Check sheet for the drawn part. Datum: minimum x, y, z corner. Units: mm. A direction names the side the tool comes from. Coordinates: 2 decimals unless noted, no trailing zeros. Loops run counter-clockwise (first coordinate to the right, second up) from the corner with the lowest first, then second, coordinate; pieces in that order, holes last. Notation, with made-up numbers: (-15.75, 70) - (12.25, 70) arc R28 cw to (12.25, 107) - close; hole circle Ø7 at (9.25, 83). An arc over 180 degrees is marked (long way). Write item = value, one per line. Start each with the question number.
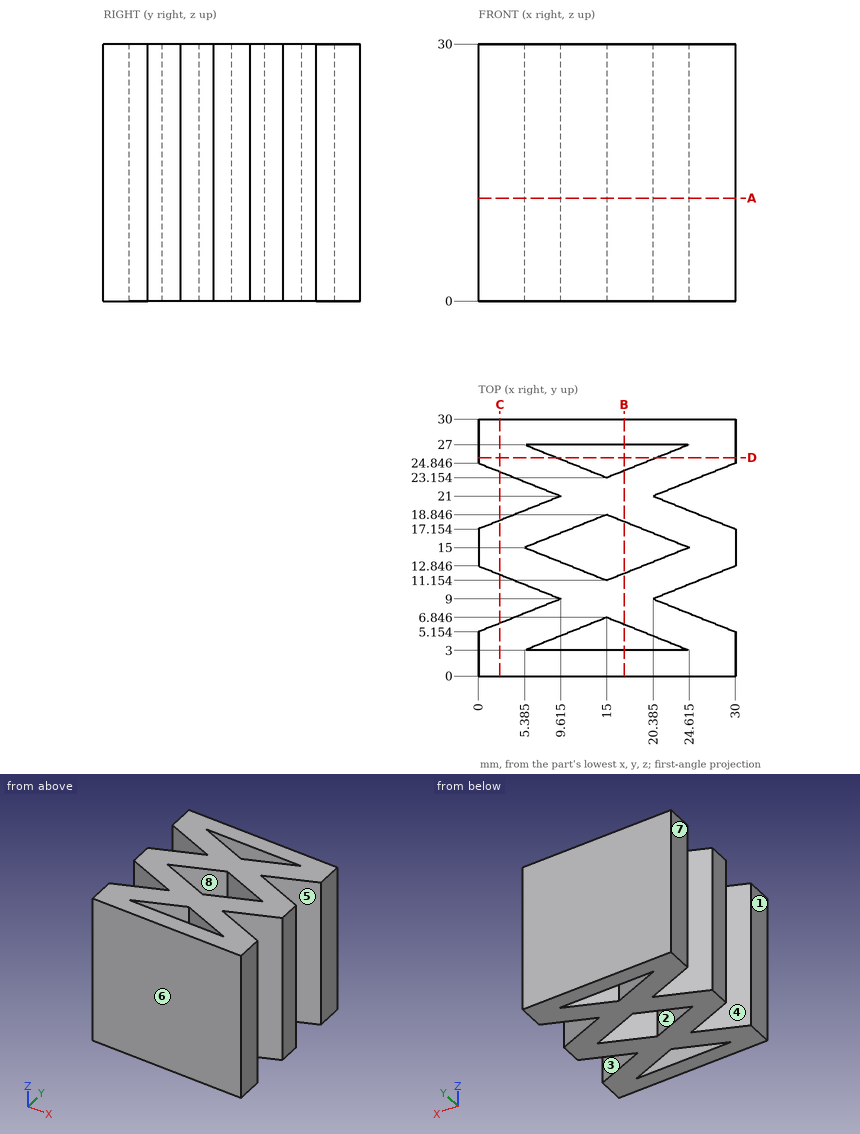
(1) Sectioned sample at D-D on y = 25.5. Enter the section's corners in (x, z) (1 decimal).
(2) Scan lines: line 1 (Y direction, x = 27, z = 4.5); line 2 (Y direction, x = 10.5, z = 3); line 3 (Y direction, x = 2, z = 2.5). Record each from-to range of solid material in increasing order.
(3) Tool access check on the marked faces 1, 2, 3 and 4. Record the directions out of +Z, -Z, +X, -X, +Y, -Y that give a thin tool (end or side, any length) a straight path to the whole face; none if there is none.
(4) Sectioned sample at C-C on x = 2.5. Enter the section's corners in (y, z).
(5) Sectioned sample at B-B on x = 17. Enter the section's corners in (y, z).
(6) Sectioned sample at A-A on z = 12. Enter the section's corners in (x, y) (1 decimal), plus the area to 3 significant figures.
(7) Draft check along Y on the marked faces 5, 6, 7 and 8. Enter one of: pulls with the +Y half, pulls with the -Y half, needs draft (parallel to the pull), parting line crosses it, or undercut.
Working result:
q1.outline = (0, 0) - (9.1, 0) - (9.1, 30) - (0, 30) - close; (20.9, 0) - (30, 0) - (30, 30) - (20.9, 30) - close
q2.line_1 = 0 to 6.35, 11.65 to 18.35, 23.65 to 30
q2.line_2 = 0 to 3, 5.05 to 12.95, 17.05 to 24.95, 27 to 30
q2.line_3 = 0 to 5.95, 12.05 to 17.95, 24.05 to 30
q3.face_1 = +Z, -Z, -X, +Y, -Y
q3.face_2 = +Z, -Z
q3.face_3 = +Z, -Z, +X
q3.face_4 = +Z, -Z, -X
q4.outline = (0, 0) - (6.15, 0) - (6.15, 30) - (0, 30) - close; (11.85, 0) - (18.15, 0) - (18.15, 30) - (11.85, 30) - close; (23.85, 0) - (30, 0) - (30, 30) - (23.85, 30) - close
q5.outline = (0, 0) - (3, 0) - (3, 30) - (0, 30) - close; (6.05, 0) - (11.95, 0) - (11.95, 30) - (6.05, 30) - close; (18.05, 0) - (23.95, 0) - (23.95, 30) - (18.05, 30) - close; (27, 0) - (30, 0) - (30, 30) - (27, 30) - close
q6.outline = (0, 0) - (30, 0) - (30, 5.2) - (20.4, 9) - (30, 12.8) - (30, 17.2) - (20.4, 21) - (30, 24.8) - (30, 30) - (0, 30) - (0, 24.8) - (9.6, 21) - (0, 17.2) - (0, 12.8) - (9.6, 9) - (0, 5.2) - close; hole (5.4, 3) - (24.6, 3) - (15, 6.8) - close; hole (5.4, 15) - (15, 11.2) - (24.6, 15) - (15, 18.8) - close; hole (5.4, 27) - (15, 23.2) - (24.6, 27) - close
q6.area = 604 mm2
q7.face_5 = undercut
q7.face_6 = pulls with the -Y half
q7.face_7 = needs draft
q7.face_8 = undercut
